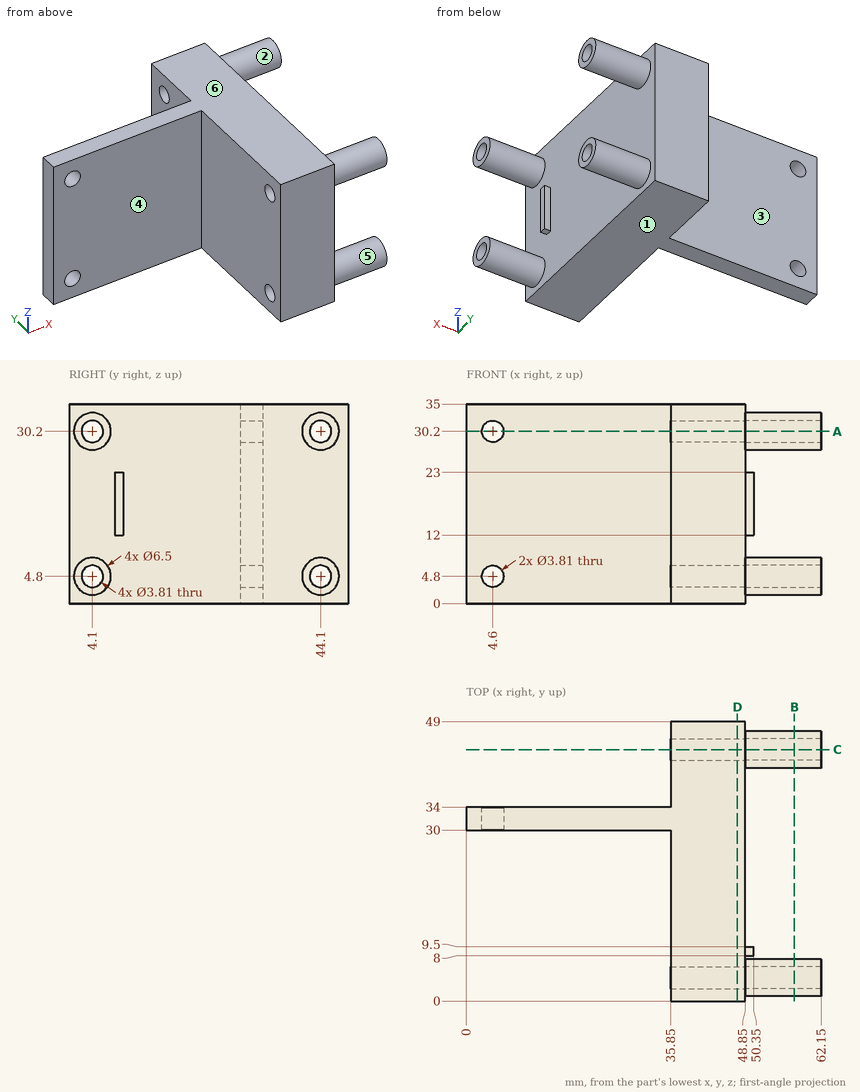
Geometry: see drawing. Coordinates: mm, zero at the bounding-box minimum. A direction names the side the tool comes from. Round coordinates to 2 decimals unless told otherwise and drop trailing zeros. Loops run counter-clockwise (first coordinate to the right, second up) from the corner with the lowest first, then second, coordinate; pieces in that order, holes last. Notation, with made-up numbers: M 81,-18 L 118,-18 A16 ccw 118,11 Z; hole C 79,-20 d4. An arc over 180 degrees is marked long. Use a Markdown table: item, result. Add a question column.
1. Section query D-D on x = 47.5. Return the cut outline in (y, z) (3 decimals).
2. Section query C-C on y = 44.1. Return the cut outline in (x, z) (3 decimals).
3. Line query: line 1 (Y direction, x = 44.25, z = 30.2) (3 decimals); line 2 (Y direction, x = 56.75, z = 30.2) (3 decimals); line 3 (Z direction, x = 49.5, y = 3). Output: solid intervals per line, ascending.
4. Section query B-B on x = 57.5. Return the cut outline in (y, z) (3 decimals).
5. Section query A-A on z = 30.2. Return the cut outline in (x, y) (3 decimals).
6. Contact query for flat-ended pins moving along their axis: P1, Ø4, axis at x = 32.5, z = 25, coming from the -Y side; P2, Ø9, axis at y = 11, z = 13.5, coming from the -X side; P3, Ø12, axis at y = 13, z = 20.5, coming from the +X side. Output: stop coordinate, or through.
7. Reachability of the marked faces 4, 5 and 6 from +Z, -Z, +X, -X, +Y, -Y: full face, straight path, thin tool, end or side. Return the list, or none.
8. Mould query, pull axis Z, two halves, no side actions, for the marked faces 1, 2 and 3. Classes: pulls with the +Z half, pulls with the -Z half, needs draft (parallel to the pull), parting line crosses it, or undercut.
Reported:
| question | item | result |
|---|---|---|
| 1 | outline | M 0,0 L 49,0 L 49,35 L 0,35 Z; hole C 4.1,4.8 d3.81; hole C 4.1,30.2 d3.81; hole C 44.1,4.8 d3.81; hole C 44.1,30.2 d3.81 |
| 2 | outline | M 35.85,0 L 48.85,0 L 48.85,1.55 L 62.15,1.55 L 62.15,2.895 L 35.85,2.895 Z; M 35.85,6.705 L 62.15,6.705 L 62.15,8.05 L 48.85,8.05 L 48.85,26.95 L 62.15,26.95 L 62.15,28.295 L 35.85,28.295 Z; M 35.85,32.105 L 62.15,32.105 L 62.15,33.45 L 48.85,33.45 L 48.85,35 L 35.85,35 Z |
| 3 | line 1 | y = 0 to 2.195, 6.005 to 42.195, 46.005 to 49 |
| 3 | line 2 | y = 0.85 to 2.195, 6.005 to 7.35, 40.85 to 42.195, 46.005 to 47.35 |
| 3 | line 3 | z = 1.74 to 3.24, 6.36 to 7.86, 27.14 to 28.64, 31.76 to 33.26 |
| 4 | outline | C 4.1,4.8 d6.5; C 4.1,30.2 d6.5; C 44.1,4.8 d6.5; C 44.1,30.2 d6.5; hole C 4.1,4.8 d3.81; hole C 4.1,30.2 d3.81; hole C 44.1,4.8 d3.81; hole C 44.1,30.2 d3.81 |
| 5 | outline | M 0,30 L 2.695,30 L 2.695,34 L 0,34 Z; M 6.505,30 L 35.85,30 L 35.85,6.005 L 62.15,6.005 L 62.15,7.35 L 48.85,7.35 L 48.85,40.85 L 62.15,40.85 L 62.15,42.195 L 35.85,42.195 L 35.85,34 L 6.505,34 Z; M 35.85,0 L 48.85,0 L 48.85,0.85 L 62.15,0.85 L 62.15,2.195 L 35.85,2.195 Z; M 35.85,46.005 L 62.15,46.005 L 62.15,47.35 L 48.85,47.35 L 48.85,49 L 35.85,49 Z |
| 6 | P1 | stops at y = 30 |
| 6 | P2 | stops at x = 35.85 |
| 6 | P3 | stops at x = 50.35 |
| 7 | face 4 | +Z, -Z, -X, -Y |
| 7 | face 5 | +X |
| 7 | face 6 | +Z, +X, -X, +Y, -Y |
| 8 | face 1 | pulls with the -Z half |
| 8 | face 2 | undercut |
| 8 | face 3 | needs draft |
